Autodesk Inventor part; units mm, degrees
ref_plane "YZ Plane" through (0, 0, 0) normal (1, 0, 0) x (0, 1, 0)
ref_plane "XZ Plane" through (0, 0, 0) normal (0, 1, 0) x (-1, 0, 0)
ref_plane "XY Plane" through (0, 0, 0) normal (0, 0, 1) x (1, 0, 0)
sketch "Sketch1" plane through (0, 0, 0) normal (0, 0, 1) x (1, 0, 0)
  line L0 (0, 0) -> (59.5, 0)
  line L1 (59.5, 0) -> (59.5, 15.4)
  line L2 (59.5, 15.4) -> (0, 15.4)
  line L3 (0, 15.4) -> (0, 0)
  line L4 (1.6, 13.8) -> (57.9, 13.8)
  line L5 (57.9, 13.8) -> (57.9, 1.6)
  line L6 (57.9, 1.6) -> (1.6, 1.6)
  line L7 (1.6, 1.6) -> (1.6, 13.8)
  dimension "d0" = 59.5
  dimension "d1" = 15.4
  dimension "d2" = 1.6
extrude "Extrusion1" add sketch "Sketch1" along normal blind 20
sketch "Sketch2" plane through (0, 0, 0) normal (0, -1, 0) x (1, 0, 0)
  line L0 (1.6, 0) -> (57.9, 0)
  line L1 (7.6, 0) -> (9.2, 0)
  line L2 (9.2, 0) -> (9.2, 14)
  line L3 (9.2, 14) -> (7.6, 14)
  line L4 (7.6, 14) -> (7.6, 0)
  line L5 (0, 0) -> (0, 20)
  dimension "d5" = 1.6
  dimension "d6" = 14
  dimension "d7" = 7.6
extrude "Extrusion2" cut sketch "Sketch2" against normal up to surface (15.4 mm away)
sketch "Sketch3" plane through (0, 0, 20) normal (0, -1, 0) x (1, 0, 0)
  line L0 (9.2, -6) -> (9.2, -20)
  line L1 (9.2, -20) -> (59.5, -20)
  line L2 (59.5, -20) -> (59.5, 0)
  line L3 (0, 0) -> (59.5, 0)
  line L4 (0, -20) -> (0, 0)
  line L5 (0, -20) -> (7.6, -20)
  line L6 (7.6, -20) -> (7.6, -6)
  line L7 (7.6, -6) -> (9.2, -6)
  line L8 (57.9, -20) -> (9.2, -20)
  line L9 (25.2, -20) -> (59.5, -20)
  line L10 (59.5, -20) -> (59.5, -6)
  line L11 (59.5, -6) -> (25.2, -6)
  line L12 (25.2, -6) -> (25.2, -20)
  dimension "d10" = 14
  dimension "d11" = 16
extrude "Extrusion3" cut sketch "Sketch3" against normal up to surface (15.4 mm away) contours L12 L11 L2 L1
sketch "Sketch4" plane through (0, 0, 20) normal (0, -1, 0) x (1, 0, 0)
  line L0 (25.2, -6) -> (59.5, -6)
  line L1 (59.5, -6) -> (59.5, 0)
  line L2 (0, 0) -> (59.5, 0)
  line L3 (0, -20) -> (0, 0)
  line L4 (0, -20) -> (7.6, -20)
  line L5 (7.6, -20) -> (7.6, -6)
  line L6 (7.6, -6) -> (9.2, -6)
  line L7 (9.2, -6) -> (9.2, -20)
  line L8 (9.2, -20) -> (25.2, -20)
  line L9 (25.2, -20) -> (25.2, -6)
  line L10 (59.5, 0) -> (54.8, 0)
  line L11 (54.8, 0) -> (54.8, -1.6)
  line L12 (54.8, -1.6) -> (59.5, -1.6)
  line L13 (59.5, -1.6) -> (59.5, 0)
  line L14 (57.9, 0) -> (1.6, 0)
  line L15 (30.8, 0) -> (26.1, 0)
  line L16 (26.1, 0) -> (26.1, -1.6)
  line L17 (26.1, -1.6) -> (30.8, -1.6)
  line L18 (30.8, -1.6) -> (30.8, 0)
  dimension "d14" = 4.7
  dimension "d15" = 1.6
  dimension "d16" = 1.6
  dimension "d17" = 4.7
  dimension "d18" = 24
extrude "Extrusion4" add sketch "Sketch4" against normal up to next contours L12 L11 L2 L1 | L18 L17 L16 L2
sketch "Sketch6" plane through (0, 0, 20) normal (0, 0, 1) x (1, 0, 0)
  line L0 (0, 0) -> (59.5, 0)
  line L1 (59.5, 0) -> (59.5, 15.4)
  line L2 (59.5, 15.4) -> (0, 15.4)
  line L3 (0, 15.4) -> (0, 0)
  line L4 (26.1, 1.6) -> (26.1, 13.8)
  line L5 (26.1, 1.6) -> (1.6, 1.6)
  line L6 (1.6, 1.6) -> (1.6, 13.8)
  line L7 (1.6, 13.8) -> (26.1, 13.8)
  line L8 (54.8, 1.6) -> (30.8, 1.6)
  line L9 (30.8, 1.6) -> (30.8, 13.8)
  line L10 (30.8, 13.8) -> (54.8, 13.8)
  line L11 (54.8, 1.6) -> (54.8, 13.8)
  line L12 (26.1, 1.6) -> (30.8, 13.8)
  line L13 (30.8, 1.6) -> (26.1, 13.8)
  line L14 (54.8, 1.6) -> (59.5, 1.6)
  line L15 (59.5, 0) -> (59.5, 15.4)
  line L16 (54.8, 13.8) -> (59.5, 13.8)
  line L17 (54.8, 1.6) -> (59.5, 13.8)
  line L18 (54.8, 13.8) -> (59.5, 1.6)
  circle A0 centre (28.45, 7.7) radius 0.85
  circle A1 centre (57.15, 7.7) radius 0.85
  point P0 (0, 0)
  dimension "d24" = 1.7
  dimension "d25" = 1.7
extrude "Extrusion5" cut sketch "Sketch6" against normal up to next contours A1 L17 L18 | L18 L17 A1 | L17 L18 A1 | A1 L18 L17 | A0 L12 L13 | L13 L12 A0 | L12 L13 A0 | L12 A0 L13
sketch "Sketch7" plane through (0, 0, 20) normal (0, -1, 0) x (1, 0, 0)
  line L0 (59.5, -6) -> (59.5, 0)
  line L1 (0, 0) -> (59.5, 0)
  line L2 (0, -20) -> (0, 0)
  line L3 (0, -20) -> (7.6, -20)
  line L4 (7.6, -20) -> (7.6, -6)
  line L5 (7.6, -6) -> (9.2, -6)
  line L6 (9.2, -6) -> (9.2, -20)
  line L7 (9.2, -20) -> (25.2, -20)
  line L8 (25.2, -20) -> (25.2, -6)
  line L9 (25.2, -6) -> (59.5, -6)
  line L10 (25.2, -6) -> (17.1171, -20)
  line L11 (9.2, -20) -> (25.2, -20)
  line L12 (25.2, -6) -> (41.3658, -6) construction
  line L13 (17.1171, -20) -> (25.2, -20)
  line L14 (25.2, -20) -> (25.2, -6)
  dimension "d28" = 120
extrude "Extrusion6" cut sketch "Sketch7" against normal up to surface (15.4 mm away) contours L8 L7 L10
properties part number "CarCab"
Could you check a few things on this model? Use its own coordinates, in mm. A direction names the side the tool comes from. Coordinates: 2 decimals unless noted, no trailing zeros. Write each loop counter-clockwise with the first axis right and the second up, starting at its lowest first coordinate (ties: lowest second). Pieces come first, ordered by that corner, then holes. Notation, with made-up numbers: (23, 39) -> (27, 39) arc R13 ccw to (27, 59) -> close; hole circle Ø2 at (-3, 55.25). An arc over 180 degrees is marked (long way). Write item = value, one per line. Start each with the question number.
(1) I want a section at C-C (y = 9.25). Please give me the cut outline in (x, z), plus the area to 3 significant figures.
(2) I want a section at B-B (z = 15.75). Please give me the cut outline in (x, y).
(3) I want a section at D-D (z = 7). Please give me the cut outline in (x, y).
(4) We'd pull the mould along Y, two halves only. Please class faces 6 (the face through (26.1, 8, 19)), 7 (the face through (59.5, 8, 17)), 8 (the face through (23.6, 15.4, 12.1)): released by +Y, released by -Y, zero draft, split by the parting line, or undercut.
(5) I need wall thicknesses on line 1 (X direction, y = 7.7, z = 19.05); line 2 (X direction, y = 7.7, z = 16.8); line 3 (Y direction, x = 6, z = 16). Which ranges of each line are inside material? Lowest first, please. Write a range as [from, to].
(6) Will these pins go through, and if not, where does the flat tip stop? pin 1 (0.5 mm diameter, centred on y = 14.5, z = 9.5, fed in from +X); pin 2 (5 mm diameter, centred on x = 29, y = 10.5, fed in from -Z); pin 3 (3.5 mm diameter, centred on y = 5, z = 9, fed in from +X).
(7) Which directions (+Z, -Z, +X, -X, +Y, -Y) give clear straight access to the entire face, cutting with the end or side of a thin tool? Please do faces 1 (the face through (23, 0, 12)), 2 (the face through (54.8, 8, 19)), 3 (the face through (45, 14, 14)), 4 (the face through (56, 8, 18.4)), 5 (the face through (9.2, 15, 7)).
(8) I want a section at A-A (x = 28.45). Please give me the cut outline in (y, z).
Result set:
q1.outline = (0, 0) -> (1.6, 0) -> (1.6, 20) -> (0, 20) -> close; (26.1, 18.4) -> (30.8, 18.4) -> (30.8, 20) -> (26.1, 20) -> close; (54.8, 18.4) -> (57.9, 18.4) -> (57.9, 14) -> (59.5, 14) -> (59.5, 20) -> (54.8, 20) -> close
q1.area = 54.1 mm2
q2.outline = (0, 0) -> (59.5, 0) -> (59.5, 15.4) -> (0, 15.4) -> close; hole (1.6, 1.6) -> (57.9, 1.6) -> (57.9, 7.3) arc R0.85 ccw to (57.9, 8.1) -> (57.9, 13.8) -> (1.6, 13.8) -> close
q3.outline = (0, 0) -> (7.6, 0) -> (7.6, 1.6) -> (1.6, 1.6) -> (1.6, 13.8) -> (7.6, 13.8) -> (7.6, 15.4) -> (0, 15.4) -> close; (9.2, 0) -> (21.16, 0) -> (21.16, 1.6) -> (9.2, 1.6) -> close; (9.2, 13.8) -> (21.16, 13.8) -> (21.16, 15.4) -> (9.2, 15.4) -> close
q4.face_6 = undercut
q4.face_7 = zero draft
q4.face_8 = released by +Y
q5.line_1 = [0, 1.6], [26.1, 27.6], [29.3, 30.8], [54.8, 56.3], [58, 59.5]
q5.line_2 = [0, 1.6], [58, 59.5]
q5.line_3 = [0, 1.6], [13.8, 15.4]
q6.pin_1 = 22.75
q6.pin_2 = 18.4
q6.pin_3 = 1.6
q7.face_1 = +Z, -Z, +X, -X, -Y
q7.face_2 = +Z, -Z
q7.face_3 = -Z, +X, +Y, -Y
q7.face_4 = -Z
q7.face_5 = -Z, +Y, -Y
q8.outline = (0, 14) -> (1.6, 14) -> (1.6, 18.4) -> (6.85, 18.4) -> (6.85, 20) -> (0, 20) -> close; (8.55, 18.4) -> (13.8, 18.4) -> (13.8, 14) -> (15.4, 14) -> (15.4, 20) -> (8.55, 20) -> close
